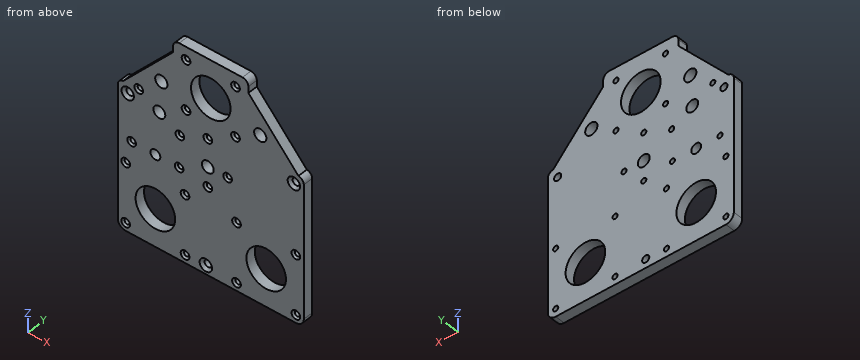
from build123d import *

# Parameters (mm, degrees)
SKETCH1_W                                       = 94
SKETCH1_H                                       = 108
BOSS_EXTRUDE1_DEPTH                             = 5
FILLET1_R                                       = 4
SKETCH22_W                                      = 28
SKETCH22_H                                      = 5
CUT_EXTRUDE3_DEPTH                              = 34
CSK_FOR_M3_FLAT_HEAD_MACHINE_SCREW1_D           = 3.6
CSK_FOR_M3_FLAT_HEAD_MACHINE_SCREW1_CSINK_D     = 6.3
CSK_FOR_M3_FLAT_HEAD_MACHINE_SCREW1_CSINK_ANGLE = 90
FILLET4_R                                       = 3
CHAMFER3_DEPTH                                  = 5
CSK_FOR_M2_FLAT_HEAD_MACHINE_SCREW2_D           = 2.6
CSK_FOR_M2_FLAT_HEAD_MACHINE_SCREW2_CSINK_D     = 4.4
CSK_FOR_M2_FLAT_HEAD_MACHINE_SCREW2_CSINK_ANGLE = 90
CUT_EXTRUDE4_DEPTH                              = 72.763500472
CUT_EXTRUDE4_DEPTH_BACK                         = 72.763500472
SKETCH25_R                                      = 1.3
SKETCH25_R_2                                    = 3
CHAMFER1_SIZE                                   = 0.9
SKETCH26_R                                      = 2.5
SKETCH26_R_2                                    = 1.3
CUT_EXTRUDE8_DEPTH                              = 10
CHAMFER2_SIZE                                   = 0.9
SKETCH27_R                                      = 10
CUT_EXTRUDE9_DEPTH                              = 10
SKETCH29_R                                      = 3.1
CUT_EXTRUDE11_DEPTH                             = 72.763500472
SKETCH30_R                                      = 3
SKETCH30_R_2                                    = 1.3
CUT_EXTRUDE12_DEPTH                             = 72.763500472
CHAMFER4_SIZE                                   = 0.9


with BuildPart() as part:
    # Sketch1 → Boss-Extrude1 (new body)
    with BuildSketch(Plane(origin=(0, 0, 0), x_dir=(1, 0, 0), z_dir=(0, 1, 0))):
        Rectangle(SKETCH1_W, SKETCH1_H)
    extrude(amount=BOSS_EXTRUDE1_DEPTH)

    # Fillet1
    fillet1_edges = [part.edges().sort_by_distance(p)[0] for p in [
        (47, 2.5, 54),
        (-47, 2.5, 54),
        (-47, 2.5, -54),
        (47, 2.5, -54),
    ]]
    fillet(fillet1_edges, radius=FILLET1_R)

    # Sketch22 → Cut-Extrude3 (cut)
    with BuildSketch(Plane.XY.offset(54)):
        with Locations((-33, 2.5)):
            Rectangle(SKETCH22_W, SKETCH22_H)
        with Locations((33, 2.5)):
            Rectangle(SKETCH22_W, SKETCH22_H)
    extrude(amount=-CUT_EXTRUDE3_DEPTH, mode=Mode.SUBTRACT)

    # CSK for M3 Flat Head Machine Screw1 (through all)
    with Locations(Plane(origin=(0, 0, 0), x_dir=(-1, 0, 0), z_dir=(0, -1, 0))):
        with Locations((-42, -49), (2.5, 49.5), (42, -49), (-42, -15), (42, -15)):
            CounterSinkHole(CSK_FOR_M3_FLAT_HEAD_MACHINE_SCREW1_D / 2, CSK_FOR_M3_FLAT_HEAD_MACHINE_SCREW1_CSINK_D / 2, counter_sink_angle=CSK_FOR_M3_FLAT_HEAD_MACHINE_SCREW1_CSINK_ANGLE)

    # Fillet4
    fillet4_edges = [part.edges().sort_by_distance(p)[0] for p in [
        (-47, 2.5, 20),
        (-19, 2.5, 54),
        (47, 2.5, 20),
        (19, 2.5, 54),
    ]]
    fillet(fillet4_edges, radius=FILLET4_R)

    # Chamfer3: read off the stored shape, not the designer's step
    # Chamfer3 outline → Chamfer3 (add)
    with BuildSketch(Plane(origin=(0, 0, 0), x_dir=(1, 0, 0), z_dir=(0, 1, 0))):
        with BuildLine():
            Line((19, -20), (19, -47.854497241))
            Line((19, -47.854497241), (44.290322581, -19.985919088))
            ThreePointArc((44.290322581, -19.985919088), (44.145331925, -19.996477704), (44, -20))
            Line((44, -20), (19, -20))
        make_face()
        with BuildLine():
            ThreePointArc((-44, -20), (-44.145331925, -19.996477704), (-44.290322581, -19.985919088))
            Line((-44.290322581, -19.985919088), (-19, -47.854497241))
            Line((-19, -47.854497241), (-19, -20))
            Line((-19, -20), (-44, -20))
        make_face()
    extrude(amount=CHAMFER3_DEPTH)

    # CSK for M2 Flat Head Machine Screw2 (through all)
    with Locations(Plane(origin=(0, 0, 0), x_dir=(-1, 0, 0), z_dir=(0, -1, 0))):
        with Locations((12.5, -47.5), (-12.5, -47.5), (12.5, -22.5), (-12.5, -22.5), (-43, 50), (-13, 50), (-43, 20), (-13, 20), (43, 50), (43, 20), (13, 50), (13, 20)):
            CounterSinkHole(CSK_FOR_M2_FLAT_HEAD_MACHINE_SCREW2_D / 2, CSK_FOR_M2_FLAT_HEAD_MACHINE_SCREW2_CSINK_D / 2, counter_sink_angle=CSK_FOR_M2_FLAT_HEAD_MACHINE_SCREW2_CSINK_ANGLE)

    # Sketch25 → Cut-Extrude4 (cut, two sides: drawn at the far end of the back side and taken through both)
    with BuildSketch(Plane(origin=(0, 0, 0), x_dir=(1, 0, 0), z_dir=(0, 1, 0)).offset(-CUT_EXTRUDE4_DEPTH_BACK)):
        with Locations(Location((-1.5, 10, 0), (0, 0, 270))):
            Circle(SKETCH25_R)
        with Locations(Location((8.5, 0, 0), (0, 0, 270))):
            Circle(SKETCH25_R)
        with Locations(Location((-1.5, -14, 0), (0, 0, 270))):
            Circle(SKETCH25_R)
        with Locations(Location((-1.5, 0, 0), (0, 0, 270))):
            Circle(SKETCH25_R_2)
    extrude(amount=CUT_EXTRUDE4_DEPTH + CUT_EXTRUDE4_DEPTH_BACK, mode=Mode.SUBTRACT)

    # Chamfer1
    chamfer1_edges = [part.edges().sort_by_distance(p)[0] for p in [
        (-1.5, 0, -11.3),
        (8.5, 0, -1.3),
        (-1.5, 0, 12.7),
    ]]
    chamfer(chamfer1_edges, length=CHAMFER1_SIZE)

    # Sketch26 → Cut-Extrude8 (cut)
    with BuildSketch(Plane(origin=(0, 0, 0), x_dir=(1, 0, 0), z_dir=(0, 1, 0))):
        with Locations(Location((-28, 8.0125, 0), (0, 0, 270))):
            Circle(SKETCH26_R)
        with Locations(Location((-40, 8.0125, 0), (0, 0, 270))):
            Circle(SKETCH26_R_2)
        with Locations(Location((-16, 8.0125, 0), (0, 0, 90))):
            Circle(SKETCH26_R_2)
    extrude(amount=CUT_EXTRUDE8_DEPTH, mode=Mode.SUBTRACT)

    # Chamfer2
    chamfer2_edges = [part.edges().sort_by_distance(p)[0] for p in [
        (-16, 0, -6.7125),
        (-40, 0, -9.3125),
    ]]
    chamfer(chamfer2_edges, length=CHAMFER2_SIZE)

    # Sketch27 → Cut-Extrude9 (cut)
    with BuildSketch(Plane(origin=(0, 5, 0), x_dir=(1, 0, 0), z_dir=(0, 1, 0))):
        with Locations(Location((-28, 35, 0), (0, 0, 270))):
            Circle(SKETCH27_R)
        with Locations(Location((28, 35, 0), (0, 0, 270))):
            Circle(SKETCH27_R)
        with Locations(Location((0, -35, 0), (0, 0, 270))):
            Circle(SKETCH27_R)
    extrude(amount=-CUT_EXTRUDE9_DEPTH, mode=Mode.SUBTRACT)

    # Sketch29 → Cut-Extrude11 (cut, through all)
    with BuildSketch(Plane(origin=(0, 5, 0), x_dir=(1, 0, 0), z_dir=(0, 1, 0))):
        with Locations(Location((-25, -30, 0), (0, 0, 270))):
            Circle(SKETCH29_R)
        with Locations(Location((25, -30, 0), (0, 0, 270))):
            Circle(SKETCH29_R)
    extrude(amount=-CUT_EXTRUDE11_DEPTH, mode=Mode.SUBTRACT)

    # Sketch30 → Cut-Extrude12 (cut, through all)
    with BuildSketch(Plane(origin=(0, 5, 0), x_dir=(1, 0, 0), z_dir=(0, 1, 0))):
        with Locations(Location((-26, -14.21, 0), (0, 0, 270))):
            Circle(SKETCH30_R)
        with Locations(Location((-15.607695155, -8.21, 0), (0, 0, 270))):
            Circle(SKETCH30_R_2)
        with Locations(Location((-36.392304845, -20.21, 0), (0, 0, 270))):
            Circle(SKETCH30_R_2)
    extrude(amount=-CUT_EXTRUDE12_DEPTH, mode=Mode.SUBTRACT)

    # Chamfer4
    chamfer4_edges = [part.edges().sort_by_distance(p)[0] for p in [
        (-36.392304845, 0, 18.91),
        (-15.607695155, 0, 6.91),
    ]]
    chamfer(chamfer4_edges, length=CHAMFER4_SIZE)


solid = part.part
Geometry: final body of the model. Coordinates: model frame, mm. Give positions to 0.01 mm unless a question says otherwise; leave off trailing zeros. Write each loop counter-clockwise with the first axis right and the second up, starting at its lowest first coordinate (ties: lowest second). Pieces come first, ordered by that corner, then holes. Notation, with made-up numbers: (71, 89.5) -> (84, 89.5) arc R8 ccw to (84, 99.5) -> close; hole circle Ø5 at (59, 36). An arc over 180 degrees is marked (long way). Answer in a Markdown table with one row per item.
(1) Section query A-A on x = -8. Return loops of the section in (y, z), then the cut area to 3 significant figures.
Answers below:
| item | result |
|---|---|
| outline | (0, -54) -> (5, -54) -> (5, 29) -> (0, 29) -> close; (0, 41) -> (5, 41) -> (5, 54) -> (0, 54) -> close |
| area | 480 mm^2 |
(2) Section query B-B on z = -35. Return loops of the section in (x, y), then the cut area to 3 significant figures.
Answers below:
| item | result |
|---|---|
| outline | (-47, 0) -> (-38, 0) -> (-38, 5) -> (-47, 5) -> close; (-18, 0) -> (18, 0) -> (18, 5) -> (-18, 5) -> close; (38, 0) -> (47, 0) -> (47, 5) -> (38, 5) -> close |
| area | 270 mm^2 |
(3) Section query C-C on y = 2.5. State how many separate pieces and enclosed holes the cut face has, then the cut area to 3 significant figures.
Answers below:
| item | result |
|---|---|
| separate pieces | 1 |
| enclosed holes | 30 |
| area | 7,730 mm^2 |
(4) Ray query, line 1 along X through (y, z) = (3.6, -35); line 2 along X through (y, z) = (4.4, -37.5); line 3 along Z through (x, y) = (-42, 2.75). Return the intervals inside material, ascending. Write a range as [from, to].
Answers below:
| item | result |
|---|---|
| line 1 | [-47, -38], [-18, 18], [38, 47] |
| line 2 | [-47, -37.68], [-18.32, 18.32], [37.68, 47] |
| line 3 | [-54, -50.83], [-49.17, -20.83], [-19.17, 13.2], [16.8, 22.51] |
(5) Pin query (flat end, axial travel): pin 1 (3.5 mm diameter, centred on x = -16, z = -8.01, fed in from -Y); pin 2 (2.5 mm diameter, centred on y = 2, z = 48.5, fed in from -X); pin 3 (3 mm diameter, centred on y = 2.5, z = 24.5, fed in from +X). Return the tip coordinate at first contact, or that it passes through.
Answers below:
| item | result |
|---|---|
| pin 1 | y = 0.45 |
| pin 2 | x = -19.55 |
| pin 3 | x = 41.56 |
